from build123d import *

# Parameters (mm, degrees)
F0_W     = 169.2275
F0_H     = 63.5
F1_DEPTH = 5.207
F2_W     = 5.207
F2_H     = 12.7
F2_W_2   = 12.7
F2_H_2   = 5.207
F2_W_3   = 18.097754
F3_DEPTH = 5.208


# Not quite as in the source:
# - a feature names something its author has since deleted; it is built from what else it names


with BuildPart() as f1:
    # F0 (on Front) → F1 (new body)
    with BuildSketch(Plane.XZ):
        Rectangle(F0_W, F0_H)
    extrude(amount=F1_DEPTH)

    # F2 (on face) → F3 (cut, through all)
    with BuildSketch(Plane(origin=(0, 0, 0), x_dir=(-1, 0, 0), z_dir=(0, 1, 0))):
        with Locations((-82.01025, 15.875)):
            Rectangle(F2_W, F2_H)
        with Locations((-82.01025, -9.525)):
            Rectangle(F2_W, F2_H)
        Polygon((-61.42101, -31.75), (-43.478704, -31.75), (-43.478704, -26.543), (-61.43371, -26.543), align=None)
        with Locations((-24.428704, -29.1465)):
            Rectangle(F2_W_2, F2_H_2)
        with Locations((0.971296, -29.1465)):
            Rectangle(F2_W_2, F2_H_2)
        with Locations((26.371296, -29.1465)):
            Rectangle(F2_W_2, F2_H_2)
        with Locations((54.470173, -29.1465)):
            Rectangle(F2_W_3, F2_H_2)
        with Locations((82.01025, 15.875)):
            Rectangle(F2_W, F2_H)
        with Locations((82.01025, -9.525)):
            Rectangle(F2_W, F2_H)
    extrude(amount=-F3_DEPTH, mode=Mode.SUBTRACT)


solid = f1.part
The model under review builds one solid part; all positions refer to its coordinate system, in mm. A direction names the side the tool comes from. Give positions to 0.01 mm unless a question says otherwise; leave off trailing zeros. Write each loop counter-clockwise with the first axis right and the second up, starting at its lowest first coordinate (ties: lowest second). Pieces come first, ordered by that corner, then holes.
1. Tool access review of faces 1 (the flat face through (25, -3, -26.543)), 2 (the flat face through (12, -3, -31.75)), 3 (the flat face through (-84.614, -3, 27)), 4 (the flat face through (-82, -3, 22.225)), 5 (the flat face through (82, -3, 9.525)): name each direction out of +Z, -Z, +X, -X, +Y, -Y from which nothing blocks a thin tool from reaching the whole face with its end or side.
2. Draft analysis for pull direction Z (two halves, no side actions). For faces 6 (the flat face through (-54, -3, -26.543)), 7 (the flat face through (-79.407, -3, 16)), 8 (the flat face through (-7.321, -3, -29)), state which applies: +Z half, -Z half, draft (parallel to the pull), parting line (faces both ways), or undercut.
3. Add section A-A, the plane z = 15.5. Write out the cut boundary in (x, y).
4. Wall thickness on L1, parallel to Z at x = 57, y = -2.55; L2, parallel to X at y = -4.3, z = 20: over which ranges is each line inside the solid? List them lowest first.
5. Add section B-B, the plane x = 23.5. Write out the cut boundary in (y, z), plus the area to 3 significant figures.
6. For P1, Ø3, axis at y = -2, z = -8.5, coming from the +X side; P2, Ø6, axis at x = 49, z = 9, coming from the +Y side; P3, Ø2.5, axis at x = 54.5, y = -3.5, coming from the -Z side; P4, Ø2.5, axis at y = -3, z = -11, coming from the -X side, all flat-tipped, find the tip position at first contact; note any pin that passes through.
Worked answers:
1. face 1: -Z, +Y, -Y
1. face 2: -Z, +X, -X, +Y, -Y
1. face 3: +Z, -Z, -X, +Y, -Y
1. face 4: -X, +Y, -Y
1. face 5: +X, +Y, -Y
2. face 6: -Z half
2. face 7: undercut
2. face 8: draft
3. outline: (-79.41, -5.21) - (79.41, -5.21) - (79.41, 0) - (-79.41, 0) - close
4. L1: z = -26.54 to 31.75
4. L2: x = -79.41 to 79.41
5. outline: (-5.21, -26.54) - (0, -26.54) - (0, 31.75) - (-5.21, 31.75) - close
5. area: 304 mm2
6. P1: stops at x = 79.41
6. P2: stops at y = 0
6. P3: stops at z = -26.54
6. P4: stops at x = -79.41
